Read the model definition and answer for the solid it produces. Units are mm, in the model's axes. A direction names the side the tool comes from. Round coordinates to 2 decimals unless told otherwise and drop trailing zeros. Order: outer loops, then holes, each group sorted by start corner. A loop starts at its lowest first (then second) coordinate and runs counter-clockwise, first axis right, second up. Notation, with made-up numbers: (-25.75, -29.5) - (25.25, -29.5) arc R11 cw to (25.25, -19.5) - close; hole circle Ø9 at (21, 29). An arc over 180 degrees is marked (long way). Put each result on its own line as item: value. Start each with the question number.
Q1. Section A-A on x = -9 is taken. State how many separate pieces and enclosed holes the cut face has, then the cut area to 3 significant figures.
Q2. Section B-B on y = -93 is taken. Give the vertices of the cut face in (x, z).
Q3. Section C-C on z = -11.5 is taken. Give the vertices of the cut face in (x, y).
Q4. Each of these flat-tipped pins is pushed along its axis until it touches: pin 1 Ø2 at (x, y) = (-26, -65.5) entering from -Z; pin 2 Ø8 at (x, y) = (-37, -27.5) entering from +Z; pin 3 Ø5 at (x, z) = (-24, -38) entering from +Y; pin 4 Ø1 at (x, y) = (-46, -44.5) entering from -Z. Where does it stop, or does it pass through?
Q5. Which of the six approach directions +Z, -Z, +X, -X, +Y, -Y give full straight-line access (tool end or side, diameter ignored) to faces 5 (the face through (-23.461, -29.425, -33.761)), 6 (the face through (-14.679, -43, -39)), 7 (the face through (-23.22, -51.01, -60.42)), 8 (the face through (-23.22, -60.61, -36.66))?
Q6. Find the intervals of material crossed by line 1 along Z through (x, y) = (-26.5, -82); line 2 along X through (y, z) = (-48, -46); line 3 along Z through (x, y) = (-3, -57), in increasing order. Write a range as from..to.
Q7. For a pull along Z with two mould halves and no side action, classify faces 1 (the face through (-65, -20, -29)), 2 (the face through (-32.045, 7.387, -18.284)), 3 (the face through (-16.76, -70.436, -59.075)), 4 (the face through (-14.902, -9.707, -34.54)) as pulls with the +Z half, pulls with the -Z half, needs draft (parallel to the pull), parting line crosses it, or undercut.
from build123d import *

# Parameters (mm, degrees)
SKETCH1_W           = 110
SKETCH1_H           = 65
BOSS_EXTRUDE1_DEPTH = 40
CHAMFER1_SIZE       = 50
SKETCH2_R           = 6.5
CUT_EXTRUDE1_DEPTH  = 99.212300536
CUT_EXTRUDE2_DEPTH  = 79.206210375


with BuildPart() as part:
    # Sketch1 → Boss-Extrude1 (new body)
    with BuildSketch(Plane(origin=(0, 0, 0), x_dir=(0, -0.927183855, -0.374606593), z_dir=(0, 0.374606593, -0.927183855))):
        with Locations((55, 32.5)):
            Rectangle(SKETCH1_W, SKETCH1_H)
    extrude(amount=BOSS_EXTRUDE1_DEPTH)

    # Chamfer1
    chamfer1_edges = [part.edges().sort_by_distance(p)[0] for p in [
        (-65, -94.498092134, -59.750402367),
    ]]
    chamfer(chamfer1_edges, length=CHAMFER1_SIZE)

    # Sketch2 → Cut-Extrude1 (cut, through all)
    with BuildSketch(Plane(origin=(-62.5, -57.94899091, -23.412912088), x_dir=(0.194241708, 0.180097776, -0.964279498), z_dir=(-0.707106781, -0.655617991, -0.264886862))):
        with Locations((24.302116706, 41.380596093)):
            Circle(SKETCH2_R)
        with Locations((36.115509488, 24.485515419)):
            Circle(SKETCH2_R)
        with Locations((17.709334516, 18.30387139)):
            Circle(SKETCH2_R)
        with Locations((30.072125815, 3.331851109)):
            Circle(SKETCH2_R)
        with Locations((42.43359242, 46.600709926)):
            Circle(SKETCH2_R)
    extrude(amount=-CUT_EXTRUDE1_DEPTH, mode=Mode.SUBTRACT)

    # Sketch3 → Cut-Extrude2 (cut, through all)
    with BuildSketch(Plane(origin=(0, 14.984263737, -37.087354183), x_dir=(0, -0.927183855, -0.374606593), z_dir=(0, 0.374606593, -0.927183855))):
        Polygon((45, 14.679491924), (65, 14.679491924), (75, 32), (65, 49.320508076), (45, 49.320508076), (35, 32), align=None)
    extrude(amount=-CUT_EXTRUDE2_DEPTH, mode=Mode.SUBTRACT)


solid = part.part
Findings:
1. separate pieces: 1
1. enclosed holes: 5
1. area: 3,460 mm2
2. outline: (-24.7, -37.57) - (-15, -63.46) - (0, -63.46) - (0, -37.57) - close
3. outline: (-65, -28.46) - (0, -28.46) - (0, 4.65) - (-65, 4.65) - close
4. pin 1: z = -70.01
4. pin 2: z = -9.49
4. pin 3: y = 14.98
4. pin 4: through
5. face 5: -Z
5. face 6: none
5. face 7: +Z, +Y
5. face 8: +Z
6. line 1: -59.78..-52.55, -39.16..-33.13
6. line 2: -63.26..-53.42, -6.52..0
6. line 3: -66.17..-42.98, -29.93..-23.03
7. face 1: needs draft
7. face 2: pulls with the +Z half
7. face 3: undercut
7. face 4: undercut
